Can you work these out from the model? Positions are in its coordinate system, mm. Face numbers are marked on the shaded views. A direction names the side the tool comes from. Give positions to 0.01 mm unless a question says otherwise; leave off trailing zeros. Loops run counter-clockwise (first coordinate to the right, second up) from the corner with the lowest first, then second, coordinate; pieces in that order, holes last. Notation, with made-up numbers: (-20, 84.5) -> (-15, 84.5) arc R17 ccw to (-15, 90.5) -> close; hole circle Ø8 at (-15, 66.25). An arc over 180 degrees is marked (long way). Return JSON: item names as keys, results as strings. Group by question number.
Q1. Suppose I cut it at A-A, the plane x = 10. Please give me the cut outline in (y, z), and give its area (3 significant figures).
Q2. Thinking about a two-plate mould opening in Z: for the marked faces 3, 4 and 5, which applies, pulls with the +Z half, pulls with the -Z half, needs draft (parallel to the pull), parting line crosses it, or undercut?
Q3. Which directions (+Z, -Z, +X, -X, +Y, -Y) give clear straight access to the entire face, cutting with the end or side of a thin tool? Please do the marked faces 1 and 2.
Q4. Suppose I cut it at C-C, the plane z = 14. Please give me the cut outline in (x, y).
Q5. Suppose I cut it at D-D, the plane y = 26. Please give me the cut outline in (x, z), and give its area (3 significant figures).
Q6. Suppose I cut it at B-B, the plane y = 13. Please give me the cut outline in (x, z).
Q7. Will these pins go through, and if not, where does the flat tip stop? pin 1 (4 mm diameter, centred on y = 14, z = 2, fed in from -X); pin 2 (5 mm diameter, centred on x = 6.5, z = 7.5, fed in from +Y); pin 3 (5 mm diameter, centred on x = 10, y = 23, fed in from -Z).
Q8. I need wall thicknesses on line 1 along Z through (x, y) = (10, -1.55); line 2 along Z through (x, y) = (8.75, 12). Which ranges of each line are inside material? Lowest first, please. Write a range as [from, to].
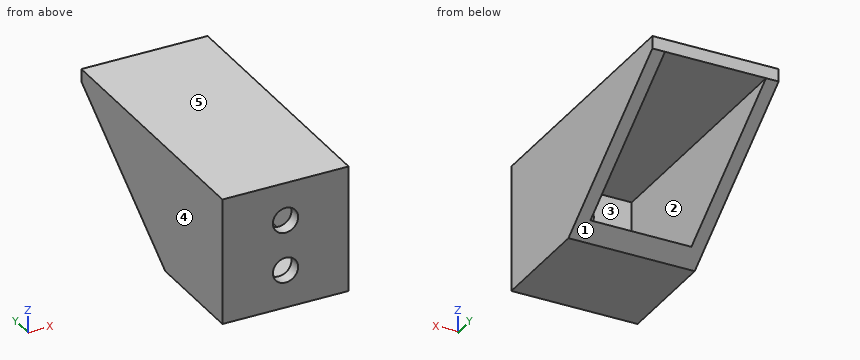
```python
from build123d import *

# Parameters (mm, degrees)
SZKIC1_W                        = 20
SZKIC1_H                        = 20
SZKIC1_W_2                      = 16
SZKIC1_H_2                      = 16
DODANIE_WYCI_GNI_CIE1_DEPTH     = 40
WYTNIJ_WYCI_GNI_CIE1_DEPTH      = 1
WYTNIJ_WYCI_GNI_CIE1_DEPTH_BACK = 21
SZKIC3_W                        = 20
SZKIC3_H                        = 20
DODANIE_WYCI_GNI_CIE2_DEPTH     = 2
SZKIC4_R                        = 2
WYTNIJ_WYCI_GNI_CIE2_DEPTH      = 2


with BuildPart() as part:
    # Szkic1 → Dodanie-wyciągnięcie1 (new body)
    with BuildSketch(Plane(origin=(0, 0, 0), x_dir=(1, 0, 0), z_dir=(0, 1, 0))):
        with Locations((10, -10)):
            Rectangle(SZKIC1_W, SZKIC1_H)
        with Locations((10, -10)):
            Rectangle(SZKIC1_W_2, SZKIC1_H_2, mode=Mode.SUBTRACT)
    extrude(amount=DODANIE_WYCI_GNI_CIE1_DEPTH)

    # Szkic2 → Wytnij-wyciągnięcie1 (cut, two sides)
    with BuildSketch(Plane(origin=(20, 0, 0), x_dir=(0, 0, -1), z_dir=(1, 0, 0))) as wytnij_wyci_gni_cie1_sk:
        Polygon((-18, 40), (0, 15), (0, 40), align=None)
    extrude(amount=WYTNIJ_WYCI_GNI_CIE1_DEPTH, mode=Mode.SUBTRACT)
    extrude(wytnij_wyci_gni_cie1_sk.sketch, amount=-WYTNIJ_WYCI_GNI_CIE1_DEPTH_BACK, mode=Mode.SUBTRACT)

    # Szkic3 → Dodanie-wyciągnięcie2 (add)
    with BuildSketch(Plane.XZ):
        with Locations((10, 10)):
            Rectangle(SZKIC3_W, SZKIC3_H)
    extrude(amount=DODANIE_WYCI_GNI_CIE2_DEPTH)

    # Szkic4 → Wytnij-wyciągnięcie2 (cut)
    with BuildSketch(Plane.XZ.offset(2)):
        with Locations((10, 14)):
            Circle(SZKIC4_R)
        with Locations((10, 6)):
            Circle(SZKIC4_R)
    extrude(amount=-WYTNIJ_WYCI_GNI_CIE2_DEPTH, mode=Mode.SUBTRACT)


solid = part.part
```
Ans:
{
 "1": {"outline": "(-2, 0) -> (15, 0) -> (17.78, 2) -> (0, 2) -> (0, 4) -> (-2, 4) -> close; (-2, 8) -> (0, 8) -> (0, 12) -> (-2, 12) -> close; (-2, 16) -> (0, 16) -> (0, 18) -> (40, 18) -> (40, 20) -> (-2, 20) -> close", "area": "137 mm^2"},
 "2": {"face 3": "undercut", "face 4": "needs draft", "face 5": "pulls with the +Z half"},
 "3": {"face 1": "-Z, +X, -X, +Y", "face 2": "+Y"},
 "4": {"outline": "(0, -2) -> (8, -2) -> (8, 0) -> (2, 0) -> (2, 34.44) -> (0, 34.44) -> close; (12, -2) -> (20, -2) -> (20, 34.44) -> (18, 34.44) -> (18, 0) -> (12, 0) -> close"},
 "5": {"outline": "(0, 7.92) -> (2, 7.92) -> (2, 18) -> (18, 18) -> (18, 7.92) -> (20, 7.92) -> (20, 20) -> (0, 20) -> close", "area": "80.3 mm^2"},
 "6": {"outline": "(0, 0) -> (20, 0) -> (20, 20) -> (0, 20) -> close; hole (2, 2) -> (18, 2) -> (18, 18) -> (2, 18) -> close"},
 "7": {"pin 1": "stops at x = 0", "pin 2": "stops at y = 0", "pin 3": "stops at z = 18"},
 "8": {"line 1": "z = [0, 4], [8, 12], [16, 20]", "line 2": "z = [0, 2], [18, 20]"}
}
